from build123d import *

# Parameters (mm, degrees)
SKETCH1_W           = 80
SKETCH1_H           = 50
BOSS_EXTRUDE1_DEPTH = 15
CUT_EXTRUDE2_DEPTH  = 10
CUT_EXTRUDE3_DEPTH  = 10
BOSS_EXTRUDE2_DEPTH = 10


with BuildPart() as part:
    # Sketch1 → Boss-Extrude1 (new body)
    with BuildSketch(Plane(origin=(0, 0, 0), x_dir=(1, 0, 0), z_dir=(0, 1, 0))):
        Rectangle(SKETCH1_W, SKETCH1_H)
    extrude(amount=BOSS_EXTRUDE1_DEPTH)

    # Sketch6 → Cut-Extrude2 (cut)
    with BuildSketch(Plane(origin=(0, 15, 0), x_dir=(1, 0, 0), z_dir=(0, 1, 0))):
        with BuildLine():
            Line((40, -15), (15, -15))
            ThreePointArc((15, -15), (0, 0), (15, 15))
            Line((15, 15), (40, 15))
            Line((40, 15), (40, -15))
        make_face()
    extrude(amount=-CUT_EXTRUDE2_DEPTH, mode=Mode.SUBTRACT)

    # Sketch8 → Cut-Extrude3 (cut)
    with BuildSketch(Plane(origin=(0, 5, 0), x_dir=(1, 0, 0), z_dir=(0, 1, 0))):
        with BuildLine():
            Line((40, -10), (15, -10))
            ThreePointArc((15, -10), (5, 0), (15, 10))
            Line((15, 10), (40, 10))
            Line((40, 10), (40, -10))
        make_face()
    extrude(amount=-CUT_EXTRUDE3_DEPTH, mode=Mode.SUBTRACT)

    # Sketch9 → Boss-Extrude2 (add)
    with BuildSketch(Plane.XY.offset(17.5)):
        Polygon((-40, 15), (-40, 50), (-24.543301065, 50), (0, 15), align=None)
    boss_extrude2 = extrude(amount=-BOSS_EXTRUDE2_DEPTH)

    # Mirror1: Boss-Extrude2 across plane
    add(boss_extrude2.mirror(Plane.XY))


solid = part.part
Verification items for the finished model (mm, model axes). A direction names the side the tool comes from. Coordinates: 2 decimals unless noted, no trailing zeros. Order: outer loops, then holes, each group sorted by start corner. A loop starts at its lowest first (then second) coordinate and runs counter-clockwise, first axis right, second up.
1. Sectioned sample at B-B, the plane y = 41. Record the cut outline in (x, z), and give its area (3 significant figures).
Results found:
outline: (-40, -17.5) - (-18.23, -17.5) - (-18.23, -7.5) - (-40, -7.5) - close; (-40, 7.5) - (-18.23, 7.5) - (-18.23, 17.5) - (-40, 17.5) - close
area: 435 mm2
2. Sectioned sample at A-A, the plane x = 22. Record the cut outline in (y, z), and give its area (3 significant figures).
Results found:
outline: (0, -25) - (15, -25) - (15, -15) - (5, -15) - (5, -10) - (0, -10) - close; (0, 10) - (5, 10) - (5, 15) - (15, 15) - (15, 25) - (0, 25) - close
area: 350 mm2
3. Sectioned sample at C-C, the plane z = -12. Record the cut outline in (x, y), and give its area (3 significant figures).
Results found:
outline: (-40, 0) - (40, 0) - (40, 5) - (6, 5) - (6, 15) - (0, 15) - (-24.54, 50) - (-40, 50) - close
area: 1,830 mm2
4. Release check for a two-part mould opening along Z. For faces 1 (the face through (28, 10, 15)), 2 (the face through (-1, 7, -25)), 3 (the face through (-32, 50, 13)) record: +Z half, -Z half, draft (parallel to the pull), parting line (faces both ways), or undercut.
Results found:
face 1: undercut
face 2: -Z half
face 3: draft
5. Sectioned sample at D-D, the plane x = -28. Record the cut outline in (y, z).
Results found:
outline: (0, -25) - (15, -25) - (15, -17.5) - (50, -17.5) - (50, -7.5) - (15, -7.5) - (15, 7.5) - (50, 7.5) - (50, 17.5) - (15, 17.5) - (15, 25) - (0, 25) - close
6. Scan lines: line 1 (Z direction, x = -20, y = 22); line 2 (Z direction, x = 33, y = 14.5); line 3 (Y direction, x = -21.5, z = 5). Record each from-to range of solid material in increasing order.
Results found:
line 1: z = -17.5 to -7.5, 7.5 to 17.5
line 2: z = -25 to -15, 15 to 25
line 3: y = 0 to 15
7. Go/stop test with flat-tipped pins: pin 1 Ø10 at (x, y) = (-13.5, 24) entering from -Z; pin 2 Ø12 at (x, y) = (27.5, 23) entering from +Z; pin 3 Ø10.5 at (x, y) = (-22, 28.5) entering from +Z; pin 4 Ø1 at (y, z) = (23.5, -11) entering from +X. Record where each tip stops, or that it passes through.
Results found:
pin 1: stops at z = -17.5
pin 2: passes through
pin 3: stops at z = 17.5
pin 4: stops at x = -5.61
8. Set-up check for faces 4 (the face through (27, 3, -10)), 5 (the face through (-24, 29, -7.5)), 6 (the face through (-24, 29, 17.5)): record each of +Z, -Z, +X, -X, +Y, -Y from which the full face is reachable in a straight line by a thin tool's end or side.
Results found:
face 4: +X, +Y, -Y
face 5: +X, -X, +Y
face 6: +Z, +X, -X, +Y
